Build history of the part. All positions in model axes, mm. Face numbers are marked on the shaded views. Round coordinates to 2 decimals unless told otherwise and drop trailing zeros. Order: outer loops, then holes, each group sorted by start corner. A loop starts at its lowest first (then second) coordinate and runs counter-clockwise, first axis right, second up. Notation, with made-up numbers: M 31.5,-12 L 77.5,-12 A7 ccw 77.5,1 Z; hole C -29.5,-8.75 d10. An arc over 180 degrees is marked long. One line per item, written item: value. Start each with the question number.
Item 1: Band-saw the part on A-A, the plane x = 0. Write the cut outline in (y, z) (3 decimals), then the cut area to 3 significant figures.
Item 2: Pin check, flat tip, straight feed: pin 1 (6 mm diameter, centred on x = -10.5, z = 33.5, fed in from +Y). Stop position of the tip, or through.
Item 3: Two-plate mould, pull along Z, no slides. Class the marked faces 1, 2 and 3: +Z half, -Z half, draft (parallel to the pull), parting line (faces both ways), or undercut.
Item 4: Band-saw the part on D-D, the plane x = 21. Write the cut outline in (y, z).
Item 5: Probe L1, parallel to X at y = 1.15, z = 21; L2, parallel to Z at x = 21, y = 1.4; L3, parallel to Z at x = 14, y = 3.8. List the from-to ranges inside material, lowest first.
Item 6: Band-saw the part on C-C, the plane z = 48. Write the cut outline in (x, y).
Item 7: Band-saw the part on B-B, the plane z = -21. Write the cut outline in (x, y), then the cut area to 3 significant figures.
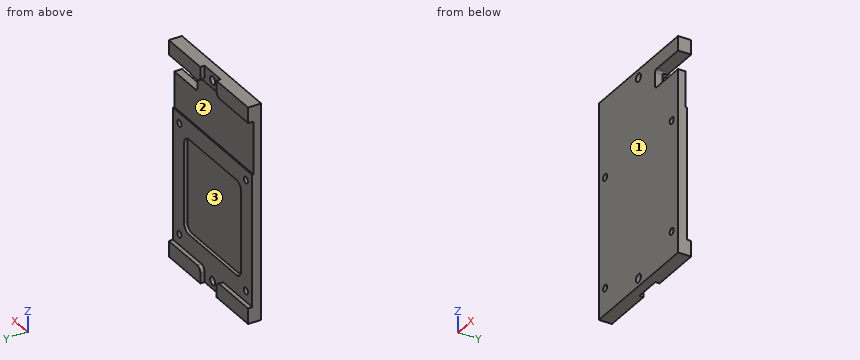
```python
from build123d import *

# Parameters (mm, degrees)
SKETCH_202_W           = 50
SKETCH_202_H           = 82
EXTRUDE_1_DEPTH        = 3.4
SKETCH_2_W             = 36.07
SKETCH_2_H             = 36.07
ADR1399KEZ_DEPTH       = 1.25
SKETCH_3_R             = 1.25
SKETCH_3_R_2           = 1.55
CUT_EXTRUDE_963_DEPTH  = 57.899560631
SKETCH_5_W             = 50
SKETCH_5_H             = 20
CUT_EXTRUDE_1417_DEPTH = 0.5
FILLET_1474_R          = 3
SKETCH_9_W             = 19.9
SKETCH_9_H             = 5.9
EXTRUDE_2_DEPTH        = 1.6
SKETCH_7_W             = 14.5
SKETCH_7_H             = 7
CUT_EXTRUDE_7_DEPTH    = 58.017541161
FILLET_3_R             = 1
FILLET_4_R             = 2


with BuildPart() as part:
    # Sketch 202 → Бобышка-Вытянуть1 (new body)
    with BuildSketch(Plane(origin=(0, 0, 0), x_dir=(1, 0, 0), z_dir=(0, 1, 0))):
        with Locations((0, -10)):
            Rectangle(SKETCH_202_W, SKETCH_202_H)
    extrude(amount=EXTRUDE_1_DEPTH)

    # Эскиз2 → Выемка для ADR1399KEZ (cut)
    with BuildSketch(Plane(origin=(0, 3.4, 0), x_dir=(1, 0, 0), z_dir=(0, 1, 0))):
        Rectangle(SKETCH_2_W, SKETCH_2_H)
    extrude(amount=-ADR1399KEZ_DEPTH, mode=Mode.SUBTRACT)

    # Эскиз3 → Cut-Extrude 963 (cut, through all)
    with BuildSketch(Plane(origin=(0, 0, 0), x_dir=(1, 0, 0), z_dir=(0, 1, 0))):
        with Locations(Location((-21, 21, 0), (0, 0, 90))):
            Circle(SKETCH_3_R)
        with Locations(Location((21, 21, 0), (0, 0, 90))):
            Circle(SKETCH_3_R)
        with Locations(Location((-21, -21, 0), (0, 0, 90))):
            Circle(SKETCH_3_R)
        with Locations(Location((21, -21, 0), (0, 0, 90))):
            Circle(SKETCH_3_R)
        with Locations(Location((0, 28, 0), (0, 0, 90))):
            Circle(SKETCH_3_R_2)
        with Locations(Location((0, -48, 0), (0, 0, 90))):
            Circle(SKETCH_3_R_2)
    extrude(amount=CUT_EXTRUDE_963_DEPTH, mode=Mode.SUBTRACT)

    # Эскиз5 → Cut-Extrude 1417 (cut)
    with BuildSketch(Plane(origin=(0, 3.4, 0), x_dir=(1, 0, 0), z_dir=(0, 1, 0))):
        with Locations((0, -35)):
            Rectangle(SKETCH_5_W, SKETCH_5_H)
    extrude(amount=-CUT_EXTRUDE_1417_DEPTH, mode=Mode.SUBTRACT)

    # Fillet 1474
    fillet_1474_edges = [part.edges().sort_by_distance(p)[0] for p in [
        (18.035, 2.775, -18.035),
        (18.035, 2.775, 18.035),
        (-18.035, 2.775, 18.035),
        (-18.035, 2.775, -18.035),
    ]]
    fillet(fillet_1474_edges, radius=FILLET_1474_R)

    # Эскиз9 → Бобышка-Вытянуть2 (add)
    with BuildSketch(Plane(origin=(0, 3.4, 0), x_dir=(1, 0, 0), z_dir=(0, 1, 0))):
        with Locations((-15.05, 28.05)):
            Rectangle(SKETCH_9_W, SKETCH_9_H)
        with Locations((15.05, 28.05)):
            Rectangle(SKETCH_9_W, SKETCH_9_H)
        with Locations((-15.05, -48.05)):
            Rectangle(SKETCH_9_W, SKETCH_9_H)
        with Locations((15.05, -48.05)):
            Rectangle(SKETCH_9_W, SKETCH_9_H)
    extrude(amount=EXTRUDE_2_DEPTH)

    # Эскиз7 → Вырез-Вытянуть7 (cut, through all)
    with BuildSketch(Plane.XZ):
        with Locations((17.75, 42)):
            Rectangle(SKETCH_7_W, SKETCH_7_H)
    extrude(amount=-CUT_EXTRUDE_7_DEPTH, mode=Mode.SUBTRACT)

    # Скругление3
    fillet_3_edges = [part.edges().sort_by_distance(p)[0] for p in [
        (10.5, 1.45, 38.5),
        (10.5, 2.5, 45.5),
    ]]
    fillet(fillet_3_edges, radius=FILLET_3_R)

    # Скругление4
    fillet_4_edges = [part.edges().sort_by_distance(p)[0] for p in [
        (5.1, 4.2, -25.1),
        (-5.1, 4.2, 45.1),
        (5.1, 4.2, 45.1),
        (-5.1, 4.2, -25.1),
    ]]
    fillet(fillet_4_edges, radius=FILLET_4_R)


solid = part.part
```
Output:
1. outline: M 0,-31 L 3.4,-31 L 3.4,-29.55 L 0,-29.55 Z; M 0,-26.45 L 3.4,-26.45 L 3.4,-18.035 L 2.15,-18.035 L 2.15,18.035 L 3.4,18.035 L 3.4,25 L 2.9,25 L 2.9,45 L 3.4,45 L 3.4,46.45 L 0,46.45 Z; M 0,49.55 L 3.4,49.55 L 3.4,51 L 0,51 Z
1. area: 203 mm²
2. pin 1: stops at y = 2.9
3. face 1: draft
3. face 2: undercut
3. face 3: undercut
4. outline: M 0,-31 L 5,-31 L 5,-25.1 L 3.4,-25.1 L 3.4,-22.25 L 0,-22.25 Z; M 0,-19.75 L 3.4,-19.75 L 3.4,19.75 L 0,19.75 Z; M 0,22.25 L 3.4,22.25 L 3.4,25 L 2.9,25 L 2.9,38.5 L 0,38.5 Z; M 0,45.5 L 5,45.5 L 5,51 L 0,51 Z
5. L1: x = -25 to -22.25, -19.75 to 19.75, 22.25 to 25
5. L2: z = -31 to -22.25, -19.75 to 19.75, 22.25 to 38.5, 45.5 to 51
5. L3: z = -31 to -25.1, 45.5 to 51
6. outline: M -25,0 L -1.55,0 L -1.55,3.4 L -5.1,3.4 L -5.1,5 L -25,5 Z; M 1.55,0 L 25,0 L 25,5 L 5.1,5 L 5.1,3.4 L 1.55,3.4 Z
7. outline: M -25,0 L -22.25,0 L -22.25,3.4 L -25,3.4 Z; M -19.75,0 L 19.75,0 L 19.75,3.4 L -19.75,3.4 Z; M 22.25,0 L 25,0 L 25,3.4 L 22.25,3.4 Z
7. area: 153 mm²
